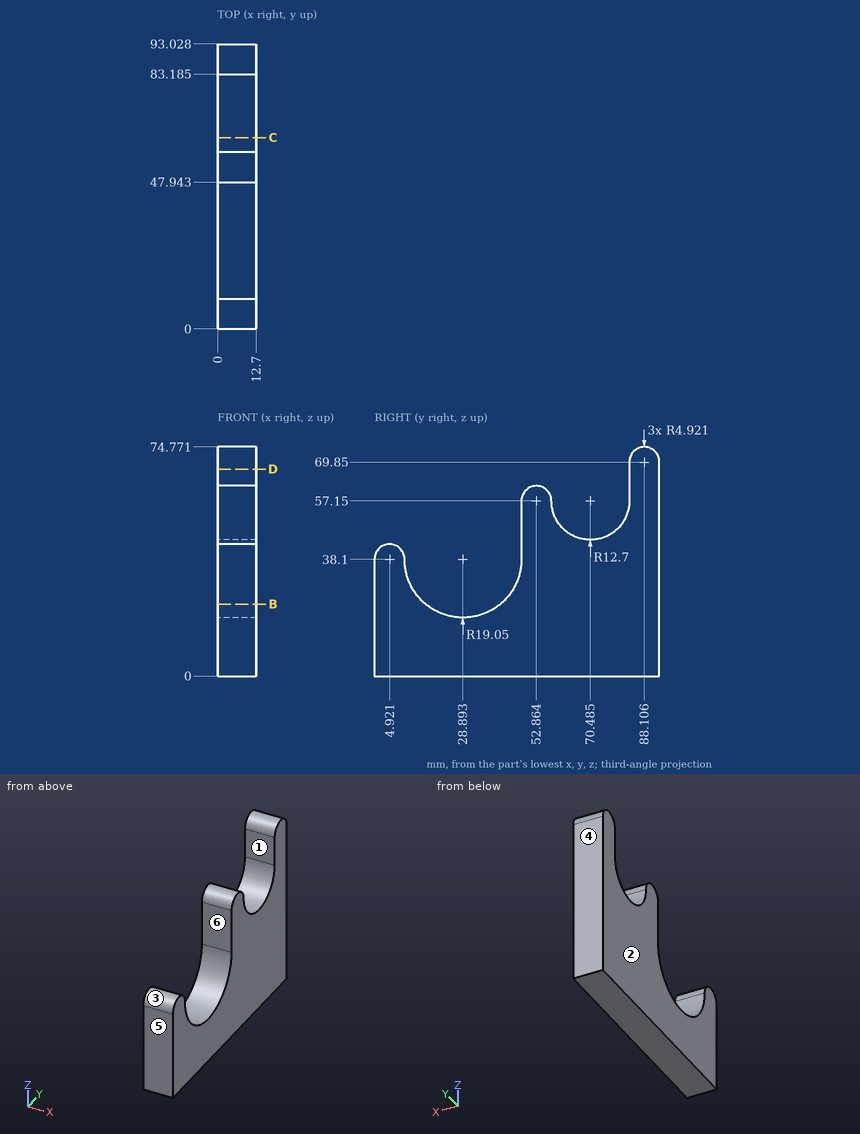
Check sheet for the drawn part. Datum: minimum x, y, z corner. Units: mm. A direction names the side the tool comes from. Give positions to 0.01 mm unless a question says otherwise; leave off trailing zeros. Write each loop counter-clockwise with the first axis right and the second up, starting at its lowest first coordinate (ties: lowest second). Pieces come first, ordered by that corner, then holes. Notation, with made-up numbers: (-34.5, 60.25) - (-30.5, 60.25) arc R17 cw to (-30.5, 64.25) - close; hole circle Ø7 at (76, -25.5). An arc over 180 degrees is marked (long way). Put each result on its own line as item: value.
1. Go/stop test with flat-tipped pins: pin 1 (2 mm diameter, centred on x = 3, y = 40.5, fed in from +Z); pin 2 (4 mm diameter, centred on x = 6, z = 46, fed in from -Y); pin 3 (4 mm diameter, centred on x = 9.5, y = 72.5, fed in from +Z). Record where each tip stops, or that it passes through.
Ans:
pin 1: stops at z = 23.82
pin 2: stops at y = 47.94
pin 3: stops at z = 45.1
2. Sectioned sample at C-C, the plane y = 62.5. Enter the section's corners in (x, z) (1 decimal).
Ans:
outline: (0, 0) - (12.7, 0) - (12.7, 47.3) - (0, 47.3) - close
3. Set-up check for the marked faces 1 and 2: record each of +Z, -Z, +X, -X, +Y, -Y from which the full face is reachable in a straight line by a thin tool's end or side.
Ans:
face 1: +Z, +X, -X
face 2: +Z, -Z, -X, +Y, -Y
4. Sectioned sample at B-B, the plane z = 23.5. Enter the section's corners in (x, y) (1 decimal).
Ans:
outline: (0, 0) - (12.7, 0) - (12.7, 16.7) - (0, 16.7) - close; (0, 41.1) - (12.7, 41.1) - (12.7, 93) - (0, 93) - close
5. Thickness scan on line 1 (Y direction, x = 1.25, z = 57.5) (1 decimal); line 2 (Y direction, x = 10, z = 52.5); line 3 (Y direction, x = 12, z = 64.5) (1 decimal). Record the ranges inside material, lowest first.
Ans:
line 1: y = 48 to 57.8, 83.2 to 93
line 2: y = 47.94 to 58.67, 82.3 to 93.03
line 3: y = 83.2 to 93
6. Draft check along Y on the marked faces 3, 4, 5 and 6. Enter one of: +Y half, -Y half, draft (parallel to the pull), parting line (faces both ways), or undercut.
Ans:
face 3: undercut
face 4: +Y half
face 5: -Y half
face 6: undercut
7. Sectioned sample at D-D, the plane z = 67.5. Enter the section's corners in (x, y) (1 decimal).
Ans:
outline: (0, 83.2) - (12.7, 83.2) - (12.7, 93) - (0, 93) - close
